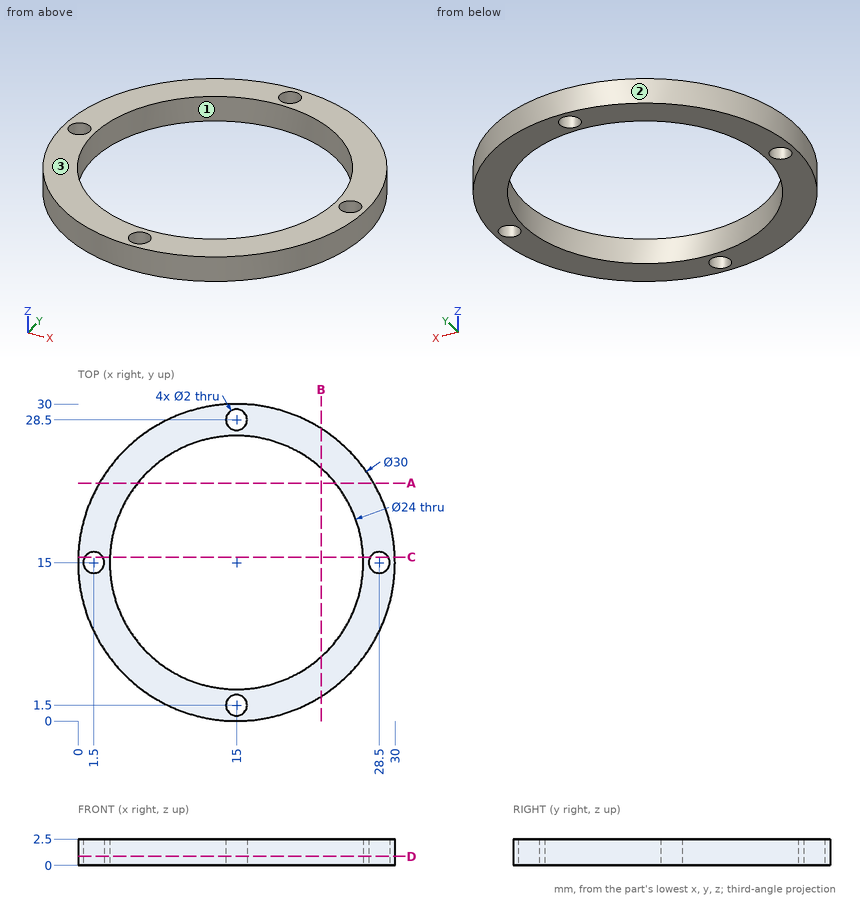
The drawing under review shows one solid part. Ordinate dimensions are in mm from its lowest x, y, z. Round coordinates to 2 decimals unless told otherwise and drop trailing zeros. Loops run counter-clockwise (first coordinate to the right, second up) from the corner with the lowest first, then second, coordinate; pieces in that order, holes last. Notation, with made-up numbers: M -5.75,-39.75 L 15.25,-39.75 A18 cw 15.25,-32.75 Z; hole C 41,12.5 d8. An arc over 180 degrees is marked long. Answer as CSV lines item,"result". Start each with the question number.
Item 1: Consider section B-B (x = 23). Write out the cut boundary in (y, z).
Item 2: Consider section C-C (y = 15.5). Write out the cut boundary in (x, z).
Item 3: Wall thickness on line 1 (Y direction, x = 15, z = 0.9); line 2 (X direction, y = 15.5, z = 0.55); line 3 (Y direction, x = 10.5, z = 1.35): over which ranges is each line inside the solid? List them lowest first. Write a range as [from, to].
Item 4: Consider section D-D (z = 0.85). Write out the cut boundary in (x, y), then the cut area to 3 significant figures.
Item 5: Insertion check: P1, Ø1.5, axis at y = 21, z = 1.5, coming from the +X side; P2, Ø1.2, axis at x = 28.5, y = 15, coming from the +Z side. Each pin has a flat end and moves straight along its axis. Give the tip position at first contact, or say it passes through.
Item 6: Mouldability with a two-part tool opening along Y and no side actions: class the marked faces 1, 2 and 3 as released by +Y, released by -Y, zero draft, split by the parting line, or undercut.
Item 7: Consider section A-A (y = 22.5). Write out the cut boundary in (x, z), then the cut area to 3 significant figures.
Answer:
1,outline,"M 2.31,0 L 6.06,0 L 6.06,2.5 L 2.31,2.5 Z; M 23.94,0 L 27.69,0 L 27.69,2.5 L 23.94,2.5 Z"
2,outline,"M 0.01,0 L 0.63,0 L 0.63,2.5 L 0.01,2.5 Z; M 2.37,0 L 3.01,0 L 3.01,2.5 L 2.37,2.5 Z; M 26.99,0 L 27.63,0 L 27.63,2.5 L 26.99,2.5 Z; M 29.37,0 L 29.99,0 L 29.99,2.5 L 29.37,2.5 Z"
3,line 1,"y = [0, 0.5], [2.5, 3], [27, 27.5], [29.5, 30]"
3,line 2,"x = [0.01, 0.63], [2.37, 3.01], [26.99, 27.63], [29.37, 29.99]"
3,line 3,"y = [0.69, 3.88], [26.12, 29.31]"
4,outline,"C 15,15 d30; hole C 1.5,15 d2; hole C 15,15 d24; hole C 15,1.5 d2; hole C 15,28.5 d2; hole C 28.5,15 d2"
4,area,"242 mm^2"
5,P1,"stops at x = 29.05"
5,P2,"passes through"
6,face 1,"undercut"
6,face 2,"split by the parting line"
6,face 3,"zero draft"
7,outline,"M 2.01,0 L 5.63,0 L 5.63,2.5 L 2.01,2.5 Z; M 24.37,0 L 27.99,0 L 27.99,2.5 L 24.37,2.5 Z"
7,area,"18.1 mm^2"
